Study the drawing (mm; zero at the part's minimum x, y, z) and answer. A direction names the side the tool comes from. Give positions to 0.01 mm unless a question says otherwise; leave off trailing zeros. Write each loop counter-clockwise with the first axis right and the second up, starting at its lowest first coordinate (ties: lowest second). Pieces come first, ordered by that corner, then holes. Notation, with made-up numbers: (-39, 69) - (-32, 69) arc R23 cw to (-32, 97) - close; hole circle Ø7 at (72, -7). An arc over 180 degrees is marked (long way). Return JSON: item names as keys, results as strings.
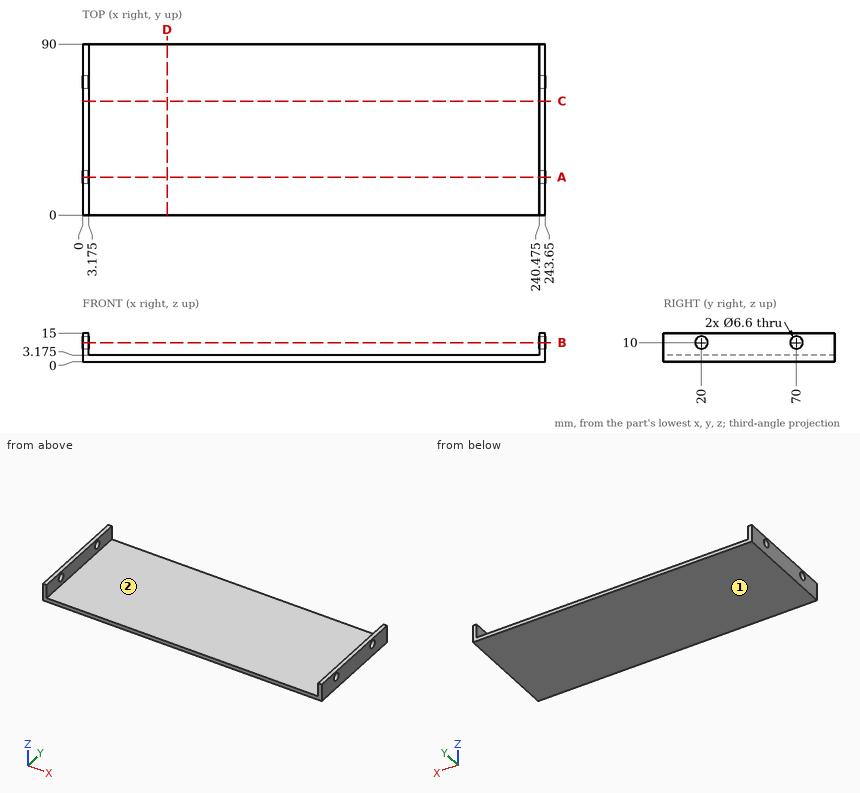
Item 1: Consider L1, parallel to Z at x = 1, y = 20; L2, parallel to X at y = 79.5, z = 4 (3 decimals); L3, parallel to Z at x = 99, y = 67 (3 decimals). Determine where each line is inside the solid, lowest interval first.
Answer below:
{"L1": "z = 0 to 6.7, 13.3 to 15", "L2": "x = 0 to 3.175, 240.475 to 243.65", "L3": "z = 0 to 3.175"}
Item 2: A cutting plane is placed at C-C on y = 60. Determine the outline of the cut face in (x, z) (3 decimals).
Answer below:
{"outline": "(0, 0) - (243.65, 0) - (243.65, 15) - (240.475, 15) - (240.475, 3.175) - (3.175, 3.175) - (3.175, 15) - (0, 15) - close"}
Item 3: A cutting plane is placed at B-B on z = 10. Determine the outline of the cut face in (x, y) (3 decimals).
Answer below:
{"outline": "(0, 0) - (3.175, 0) - (3.175, 16.7) - (0, 16.7) - close; (0, 23.3) - (3.175, 23.3) - (3.175, 66.7) - (0, 66.7) - close; (0, 73.3) - (3.175, 73.3) - (3.175, 90) - (0, 90) - close; (240.475, 0) - (243.65, 0) - (243.65, 16.7) - (240.475, 16.7) - close; (240.475, 23.3) - (243.65, 23.3) - (243.65, 66.7) - (240.475, 66.7) - close; (240.475, 73.3) - (243.65, 73.3) - (243.65, 90) - (240.475, 90) - close"}
Item 4: A cutting plane is placed at D-D on x = 44.5. Determine the outline of the cut face in (y, z) (3 decimals), then the cut area to 3 significant figures.
Answer below:
{"outline": "(0, 0) - (90, 0) - (90, 3.175) - (0, 3.175) - close", "area": "286 mm²"}
Item 5: A flat-ended cylindrical pin translates along its axis: P1, Ø8, axis at x = 212, y = 73, coming from the +Z side (3 decimals). Find the tip coordinate at first contact, or state that the pin passes through.
Answer below:
{"P1": "stops at z = 3.175"}
Item 6: For the marked faces 1 and 2, determine the directions among +Z, -Z, +X, -X, +Y, -Y from which every point of the face is accessible in a straight line to the end or side of a thin tool.
Answer below:
{"face 1": "-Z, +X, -X, +Y, -Y", "face 2": "+Z, +Y, -Y"}
Item 7: A cutting plane is placed at A-A on y = 20. Determine the outline of the cut face in (x, z) (3 decimals), then the cut area to 3 significant figures.
Answer below:
{"outline": "(0, 0) - (243.65, 0) - (243.65, 6.7) - (240.475, 6.7) - (240.475, 3.175) - (3.175, 3.175) - (3.175, 6.7) - (0, 6.7) - close; (0, 13.3) - (3.175, 13.3) - (3.175, 15) - (0, 15) - close; (240.475, 13.3) - (243.65, 13.3) - (243.65, 15) - (240.475, 15) - close", "area": "807 mm²"}
